Geometry check sheet. Reference: the model listing, model coordinates, mm. Give positions to 0.01 mm unless a question says otherwise; leave off trailing zeros. Loops run counter-clockwise (first coordinate to the right, second up) from the corner with the lowest first, then second, coordinate; pieces in that order, holes last. Notation, with made-up numbers: (80.25, -29) -> (110.25, -29) arc R16 cw to (110.25, -7) -> close; hole circle Ø1 at (82.25, 19). An arc over 180 degrees is marked (long way). One line per question, with ' | ' between items.
from build123d import *

# Parameters (mm, degrees)
SKETCH_2_W      = 300
SKETCH_2_H      = 120
SKETCH_2_R      = 1.5
SKETCH_2_R_2    = 2
SKETCH_2_R_3    = 6.9
SKETCH_2_R_4    = 7.5
SKETCH_2_W_2    = 46
SKETCH_2_H_2    = 21.5
EXTRUDE_2_DEPTH = 3
FILLET_1_R      = 20


with BuildPart() as part:
    # Эскиз2 → Бобышка-Вытянуть2 (new body)
    with BuildSketch(Plane(origin=(0, 0, 0), x_dir=(1, 0, 0), z_dir=(0, 1, 0))):
        with Locations((-150, 60)):
            Rectangle(SKETCH_2_W, SKETCH_2_H)
        with Locations((-283, 108)):
            Circle(SKETCH_2_R, mode=Mode.SUBTRACT)
        with Locations((-17, 108)):
            Circle(SKETCH_2_R_2, mode=Mode.SUBTRACT)
        with Locations((-17, 12)):
            Circle(SKETCH_2_R, mode=Mode.SUBTRACT)
        with Locations((-283, 12)):
            Circle(SKETCH_2_R, mode=Mode.SUBTRACT)
        with Locations((-168, 35.746485704)):
            Circle(SKETCH_2_R_3, mode=Mode.SUBTRACT)
        with Locations((-252, 35.746485704)):
            Circle(SKETCH_2_R_4, mode=Mode.SUBTRACT)
        with BuildLine():
            Line((-271.607074704, 34.057157396), (-265.660946054, 35.325664842))
            ThreePointArc((-265.660946054, 35.325664842), (-218.226909759, 96.396129604), (-150, 60))
            ThreePointArc((-150, 60), (-81.773090241, 23.603870396), (-34.339053946, 84.674335158))
            Line((-34.339053946, 84.674335158), (-40.302985362, 83.402029789))
            ThreePointArc((-40.302985362, 83.402029789), (-83.530907836, 29.366412701), (-144.429139855, 62.228344058))
            ThreePointArc((-144.429139855, 62.228344058), (-219.982275004, 102.154609074), (-271.607074704, 34.057157396))
        make_face(mode=Mode.SUBTRACT)
        with Locations((-207, 35.746485704)):
            Rectangle(SKETCH_2_W_2, SKETCH_2_H_2, mode=Mode.SUBTRACT)
    extrude(amount=EXTRUDE_2_DEPTH)

    # Скругление1
    fillet_1_edges = [part.edges().sort_by_distance(p)[0] for p in [
        (0, 1.5, 0),
        (-300, 1.5, 0),
        (-300, 1.5, -120),
        (0, 1.5, -120),
    ]]
    fillet(fillet_1_edges, radius=FILLET_1_R)


solid = part.part
Item 1: Sectioned sample at B-B (x = -102.5). Record the cut outline in (y, z), plus the area to 3 significant figures.
Result:
outline: (0, -120) -> (3, -120) -> (3, -28.91) -> (0, -28.91) -> close; (0, -22.85) -> (3, -22.85) -> (3, 0) -> (0, 0) -> close | area: 342 mm2
Item 2: Sectioned sample at C-C (z = -79.5). Record the cut outline in (x, y).
Result:
outline: (-300, 0) -> (-256.8, 0) -> (-256.8, 3) -> (-300, 3) -> close; (-248.77, 0) -> (-162.65, 0) -> (-162.65, 3) -> (-248.77, 3) -> close; (-154.62, 0) -> (-40.36, 0) -> (-40.36, 3) -> (-154.62, 3) -> close; (-34.36, 0) -> (0, 0) -> (0, 3) -> (-34.36, 3) -> close
Item 3: Sectioned sample at A-A (x = -255.5). Record the cut outline in (y, z), plus the area to 3 significant figures.
Result:
outline: (0, -120) -> (3, -120) -> (3, -81.04) -> (0, -81.04) -> close; (0, -71.2) -> (3, -71.2) -> (3, -42.38) -> (0, -42.38) -> close; (0, -29.11) -> (3, -29.11) -> (3, 0) -> (0, 0) -> close | area: 291 mm2
Item 4: Release check for a two-part mould opening along X. For faces 1 (the face through (-82.503, 1.479, -29.586)), 2 (the face through (-152, 3, -61)), 3 (the face through (-6.014, 1.521, -114.297)) record: pulls with the +X half, pulls with the -X half, needs draft (parallel to the pull), parting line crosses it, or undercut.
Result:
face 1: undercut | face 2: needs draft | face 3: pulls with the +X half
Item 5: Depth check by flat-ended pin: pin 1 Ø1.8 at (x, z) = (-283, -12) entering from +Y. Enter the tip coordinate at first touch or a pass-through.
Result:
pin 1: through
Item 6: Scan lines: probe 1 along Z at (x, y) = (-207, 2.5); probe 2 along Z at (x, y) = (-252, 1.9); probe 3 along X at (y, z) = (1.95, -108). Record each from-to range of solid material in increasing order.
Result:
probe 1: -120 to -103.7, -97.7 to -46.5, -25 to 0 | probe 2: -120 to -84.76, -75.89 to -43.25, -28.25 to 0 | probe 3: -298.33 to -284.5, -281.5 to -19, -15 to -1.67
Item 7: Sectioned sample at D-D (y = 1.55). Give the number of separate pieces and of enclosed holes in the cut face, plus the area to 3 significant figures.
Result:
separate pieces: 1 | enclosed holes: 8 | area: 32,300 mm2
